Job drawing, mm, ordinate dimensions from the low corner. One solid piece. A direction names the side the tool comes from. Give positions to 0.01 mm unless a question says otherwise; leave off trailing zeros. Loops run counter-clockwise (first coordinate to the right, second up) from the corner with the lowest first, then second, coordinate; pieces in that order, holes last.
Item 1: Which spindle directions (+Z, -Z, +X, -X, +Y, -Y) get a long thin tool onto all of the face, cutting with end or side? Do the marked faces 1 and 2. Say none if no direction does.
Item 2: Mould opens along Y. For the marked faces 3, 4 and 5 say: released by +Y, released by -Y, zero draft, split by the parting line, or undercut.
Item 3: Saw through at A-A on y = 42.5. Give the cut face in (x, z), plus the area to 3 significant figures.
Item 4: Saw through at B-B on z = 10. Give the cut face in (x, y), plus the area to 3 significant figures.
Item 5: Drop flat-ended pins along their axis: P1, Ø3, axis at y = 10, z = 11, coming from the +X side; P2, Ø4.5, axis at y = 42.5, z = 10, coming from the -X side. Give the stop position or say it passes through.
Item 6: Probe probe 1 along Z at (x, y) = (12, 7.5); probe 2 along Y at (x, z) = (7.25, 11.5); probe 3 along Y at (x, z) = (9.75, 13.5). List the from-to ranges inside material, lowest first.
Item 7: Saw through at C-C on x = 11.5. Give the cut face in (y, z).
Item 8: Saw through at D-D on x = 6. Give the cut face in (y, z), plus the area to 3 significant figures.
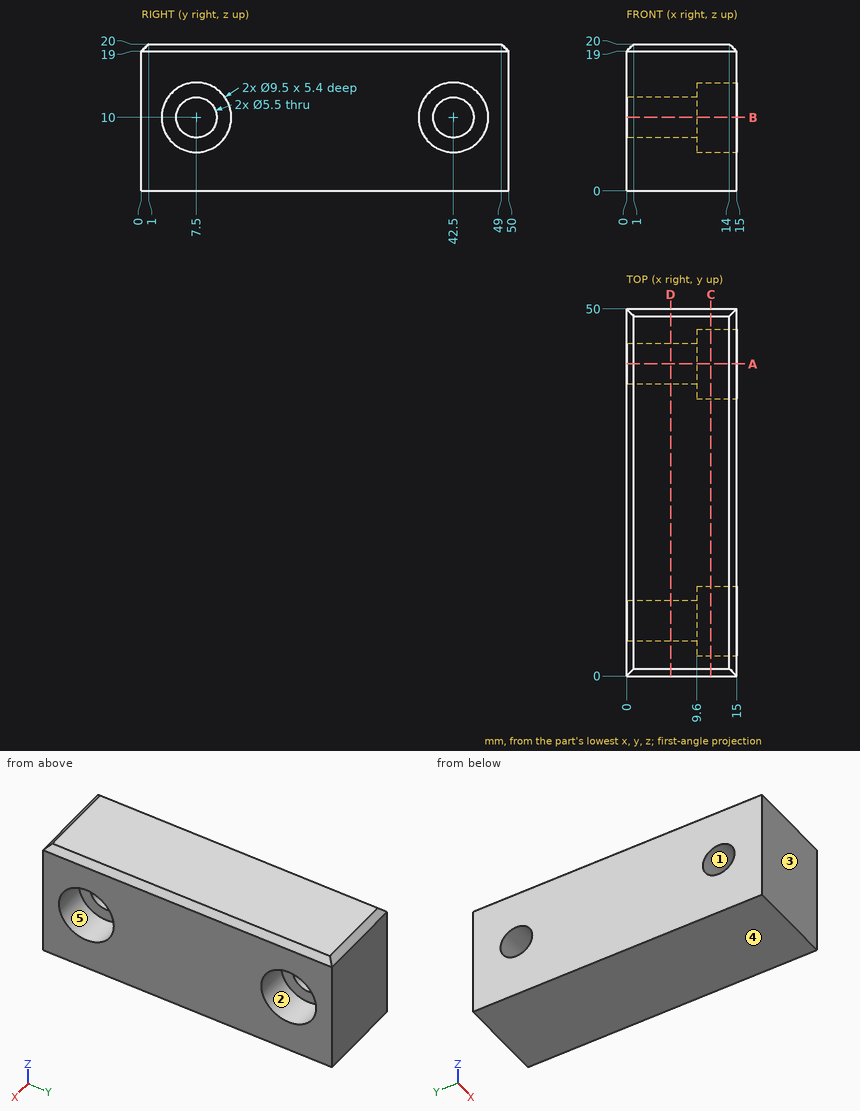
Results below:
1. face 1: +X, -X
1. face 2: +X
2. face 3: released by -Y
2. face 4: zero draft
2. face 5: undercut
3. outline: (0, 0) - (15, 0) - (15, 5.25) - (9.6, 5.25) - (9.6, 7.25) - (0, 7.25) - close; (0, 12.75) - (9.6, 12.75) - (9.6, 14.75) - (15, 14.75) - (15, 19) - (14, 20) - (1, 20) - (0, 19) - close
3. area: 195 mm2
4. outline: (0, 0) - (15, 0) - (15, 2.75) - (9.6, 2.75) - (9.6, 4.75) - (0, 4.75) - close; (0, 10.25) - (9.6, 10.25) - (9.6, 12.25) - (15, 12.25) - (15, 37.75) - (9.6, 37.75) - (9.6, 39.75) - (0, 39.75) - close; (0, 45.25) - (9.6, 45.25) - (9.6, 47.25) - (15, 47.25) - (15, 50) - (0, 50) - close
4. area: 542 mm2
5. P1: stops at x = 9.6
5. P2: passes through
6. probe 1: z = 0 to 5.25, 14.75 to 20
6. probe 2: y = 0 to 5.2, 9.8 to 40.2, 44.8 to 50
6. probe 3: y = 0 to 4.29, 10.71 to 39.29, 45.71 to 50
7. outline: (0, 0) - (50, 0) - (50, 19) - (49, 20) - (1, 20) - (0, 19) - close; hole circle Ø9.5 at (7.5, 10); hole circle Ø9.5 at (42.5, 10)
8. outline: (0, 0) - (50, 0) - (50, 19) - (49, 20) - (1, 20) - (0, 19) - close; hole circle Ø5.5 at (7.5, 10); hole circle Ø5.5 at (42.5, 10)
8. area: 951 mm2
